Work out the finished part from the listing and answer in its coordinate system (mm). Face numbers are marked on the shaded views. A direction names the side the tool comes from. Round coordinates to 2 decimals unless told otherwise and drop trailing zeros. Loops run counter-clockwise (first coordinate to the right, second up) from the corner with the lowest first, then second, coordinate; pieces in that order, holes last. Notation, with made-up numbers: M 47.5,-9 L 85.5,-9 A24 cw 85.5,8 Z; hole C 86.25,69 d10. An arc over 180 degrees is marked long. One line per item, written item: value.
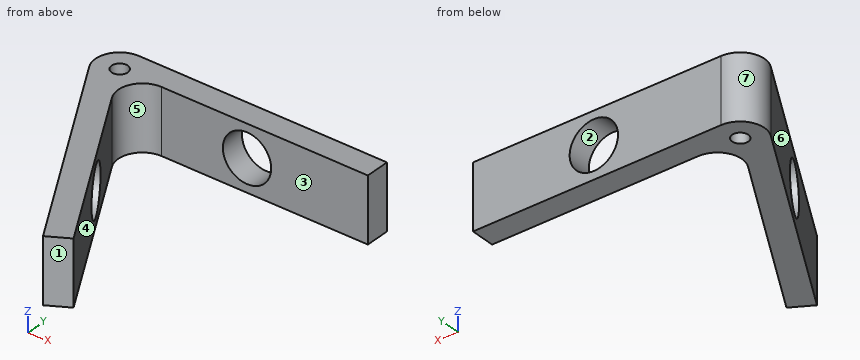
```python
from build123d import *

# Parameters (mm, degrees)
F0_R     = 2.5
F1_DEPTH = 20
F2_R     = 7.5
F3_DEPTH = 25
F4_R     = 7.5
F5_DEPTH = 25


with BuildPart() as f1:
    # F0 (on Top) → F1 (new body)
    with BuildSketch(Plane.XY):
        with BuildLine():
            Line((90, 0), (12.9903810568, 0))
            ThreePointArc((12.9903810568, 0), (6.4951905284, -3.75), (6.4951905284, -11.25))
            Line((6.4951905284, -11.25), (45, -77.9422863406))
            Line((45, -77.9422863406), (51.4951905284, -74.1922863406))
            Line((51.4951905284, -74.1922863406), (19.4855715851, -18.75))
            ThreePointArc((19.4855715851, -18.75), (19.4855715851, -11.25), (25.9807621135, -7.5))
            Line((25.9807621135, -7.5), (90, -7.5))
            Line((90, -7.5), (90, 0))
        make_face()
        with Locations((12.9903810568, -7.5)):
            Circle(F0_R, mode=Mode.SUBTRACT)
    extrude(amount=F1_DEPTH)

    # F2 (on face) → F3 (cut)
    with BuildSketch(Plane(origin=(0, 0, 0), x_dir=(0.5, -0.8660254038, 0), z_dir=(-0.8660254038, -0.5, 0))):
        with Locations((52.5, 10)):
            Circle(F2_R)
    extrude(amount=-F3_DEPTH, mode=Mode.SUBTRACT)

    # F4 (on face) → F5 (cut)
    with BuildSketch(Plane(origin=(0, 0, 0), x_dir=(-1, 0, 0), z_dir=(0, 1, 0))):
        with Locations((-52.5, 10)):
            Circle(F4_R)
    extrude(amount=-F5_DEPTH, mode=Mode.SUBTRACT)


solid = f1.part
```
1) Find section B-B (z = 8.75). Give the vertices of the cut face in (x, y), then the cut area to 3 significant figures.
Check values:
outline: M 6.5,-11.25 L 22.55,-39.06 L 29.05,-35.31 L 19.49,-18.75 A7.5 cw 25.98,-7.5 L 45.1,-7.5 L 45.1,0 L 12.99,0 A7.5 ccw Z; M 29.95,-51.87 L 45,-77.94 L 51.5,-74.19 L 36.44,-48.12 Z; M 59.9,-7.5 L 90,-7.5 L 90,0 L 59.9,0 Z; hole C 12.99,-7.5 d5
area: 1,010 mm2
2) Find section D-D (z = 13.25). Give the vertices of the cut face in (x, y), then the cut area to 3 significant figures.
Check values:
outline: M 6.5,-11.25 L 22.87,-39.61 L 29.37,-35.86 L 19.49,-18.75 A7.5 cw 25.98,-7.5 L 45.74,-7.5 L 45.74,0 L 12.99,0 A7.5 ccw Z; M 29.63,-51.32 L 45,-77.94 L 51.5,-74.19 L 36.12,-47.57 Z; M 59.26,-7.5 L 90,-7.5 L 90,0 L 59.26,0 Z; hole C 12.99,-7.5 d5
area: 1,030 mm2
3) The mould has two halves that part along Y. Classify the marked faces 4, 5, 6 and 7: +Y half, -Y half, draft (parallel to the pull), parting line (faces both ways), or undercut.
Check values:
face 4: undercut
face 5: undercut
face 6: -Y half
face 7: parting line
4) Find section A-A (z = 18.5). Give the vertices of the cut face in (x, y), then the cut area to 3 significant figures.
Check values:
outline: M 6.5,-11.25 L 45,-77.94 L 51.5,-74.19 L 19.49,-18.75 A7.5 cw 25.98,-7.5 L 90,-7.5 L 90,0 L 12.99,0 A7.5 ccw Z; hole C 12.99,-7.5 d5
area: 1,230 mm2
5) Each of these flat-tipped pins is pushed along its axis until it touches: pin 1 (12 mm diameter, centred on y = -69, z = 5, fed in from -X); pin 2 (2 mm diameter, centred on y = -52.5, z = 14.5, fed in from +X); pin 3 (5 mm diameter, centred on x = 58, z = 14, fed in from -Y). Where does it stop, or does it pass through?
Check values:
pin 1: x = 36.37
pin 2: x = 39.55
pin 3: y = -7.5
6) Find the intervals of material crossed by probe 1 along Z at (x, y) = (52.5, -3.25); probe 2 along X at (y, z) = (-6.5, 5.5); probe 3 along Y at (x, z) = (44.5, 6.25), in increasing order. Write a range as from..to.
Check values:
probe 1: 0..2.5, 17.5..20
probe 2: 5.56..10.7, 15.28..46.5, 58.5..90
probe 3: -77.08..-62.08, -7.5..0
7) For the marked faces 1, 2 and 3, determine the directions among +Z, -Z, +X, -X, +Y, -Y from which every point of the face is accessible in a straight line to the end or side of a thin tool.
Check values:
face 1: +Z, -Z, +X, -Y
face 2: +Y
face 3: +Z, -Z, +X
8) Find section C-C (x = 52.5). Give the vertices of the cut face in (y, z).
Check values:
outline: M -7.5,0 L 0,0 L 0,2.5 L -7.5,2.5 Z; M -7.5,17.5 L 0,17.5 L 0,20 L -7.5,20 Z
